```python
from build123d import *

# Parameters (mm, degrees)
SKETCH_1_R                = 45
EXTRUDE_2_DEPTH           = 25
SKETCH_2_R                = 35
CUT_EXTRUDE_1_DEPTH       = 4.5
SKETCH_3_R                = 27
CUT_EXTRUDE_2_DEPTH       = 8
SKETCH_4_R                = 18
CUT_EXTRUDE_3_DEPTH       = 8.5
SKETCH_10_R               = 42.5
CUT_EXTRUDE_5_DEPTH       = 4
HOLE_WIZARD_2_D           = 3.6
HOLE_WIZARD_2_CBORE_D     = 6
HOLE_WIZARD_2_CBORE_DEPTH = 3.4
PATTERN_CIRCULAR_2_COUNT  = 12
PATTERN_CIRCULAR_3_COUNT  = 8


with BuildPart() as part:
    # Sketch 1 → Extrude 2 (new body)
    with BuildSketch(Plane.XY):
        Circle(SKETCH_1_R)
    extrude(amount=EXTRUDE_2_DEPTH)

    # Sketch 2 → Cut-Extrude 1 (cut)
    with BuildSketch(Plane.XY.offset(25)):
        Circle(SKETCH_2_R)
    extrude(amount=-CUT_EXTRUDE_1_DEPTH, mode=Mode.SUBTRACT)

    # Sketch 3 → Cut-Extrude 2 (cut)
    with BuildSketch(Plane.XY.offset(20.5)):
        Circle(SKETCH_3_R)
    extrude(amount=-CUT_EXTRUDE_2_DEPTH, mode=Mode.SUBTRACT)

    # Sketch 4 → Cut-Extrude 3 (cut)
    with BuildSketch(Plane.XY.offset(12.5)):
        Circle(SKETCH_4_R)
    extrude(amount=-CUT_EXTRUDE_3_DEPTH, mode=Mode.SUBTRACT)

    # Sketch 10 → Cut-Extrude 5 (cut)
    with BuildSketch(Plane(origin=(0, 0, 0), x_dir=(-1, 0, 0), z_dir=(0, 0, -1))):
        Circle(SKETCH_10_R)
    extrude(amount=-CUT_EXTRUDE_5_DEPTH, mode=Mode.SUBTRACT)

    # Hole Wizard 2 (through all)
    with Locations(Plane(origin=(0, 0, 4), x_dir=(-1, 0, 0), z_dir=(0, 0, -1))):
        with Locations((0, 22)):
            hole_wizard_2 = CounterBoreHole(HOLE_WIZARD_2_D / 2, HOLE_WIZARD_2_CBORE_D / 2, HOLE_WIZARD_2_CBORE_DEPTH)

    # Pattern Circular 2: Hole Wizard 2 ×12 about axis
    pattern_circular_2_axis = Axis((0, 0, 0), (0, 0, 1))
    for i in range(1, PATTERN_CIRCULAR_2_COUNT):
        add(hole_wizard_2.rotate(pattern_circular_2_axis, i * 360 / PATTERN_CIRCULAR_2_COUNT), mode=Mode.SUBTRACT)

    # Sketch 17 → Hole Wizard M3 _1 (revolve, cut)
    with BuildSketch(Plane(origin=(0, 37.5, 4), x_dir=(0, 1, 0), z_dir=(1, 0, 0))):
        Polygon((0, 0), (0, 7.251075774), (1.25, 6.5), (1.25, 0), align=None)
    hole_wizard_m3_1 = revolve(axis=Axis((0, 37.5, -2.35), (0, 0, 1)), mode=Mode.SUBTRACT)

    # Pattern Circular 3: Hole Wizard M3 _1 ×8 about axis
    pattern_circular_3_axis = Axis((0, 0, 0), (0, 0, 1))
    for i in range(1, PATTERN_CIRCULAR_3_COUNT):
        add(hole_wizard_m3_1.rotate(pattern_circular_3_axis, i * 360 / PATTERN_CIRCULAR_3_COUNT), mode=Mode.SUBTRACT)


solid = part.part
```
Here's how the part is built. I have some questions about the finished solid (model axes, mm). A direction names the side the tool comes from. Coordinates: 2 decimals unless noted, no trailing zeros. Order: outer loops, then holes, each group sorted by start corner. A loop starts at its lowest first (then second) coordinate and runs counter-clockwise, first axis right, second up. Notation, with made-up numbers: (67, 56) - (122, 56) arc R11 ccw to (122, 77) - close; hole circle Ø2 at (85, -34.5). An arc over 180 degrees is marked (long way). One line per question, with ' | ' between items. Start each with the question number.
1. Please list where these lines run through material, in increasing order: line 1 along Y through (x, z) = (0, 5.95); line 2 along Z through (x, y) = (30, -5); line 3 along Y through (x, z) = (13, 10.5). Write a range as [from, to].
2. If we section it at B-B (y = 31): Write out the boundary of the cut face in (x, z).
3. I'm going to push flat-ended pins straight in: pin 1 Ø1.8 at (x, y) = (-19.5, 10.5) entering from -Z; pin 2 Ø6 at (x, z) = (1.5, 20) entering from +Y; pin 3 Ø6 at (x, y) = (-22, 0) entering from +Z; pin 4 Ø8 at (x, y) = (0, 22) entering from -Z. Where does each tip first touch, or does it pass through?
4. If we section it at C-C (x = 11): Give the number of separate pieces and of enclosed holes in the cut face, and give its area (3 significant figures).
5. If we mould it in two halves opening along X, with no side actions, what happens to faces 4 (the flat face through (23.1, -26.5, 25)), 5 (the cylindrical face through (-17.73, 9.78, 9.99)), 6 (the cylindrical face through (20.765, -39.923, 12.325)), 7 (the cylindrical face through (-27.094, -27.625, 7.204))? For each: released by +X, released by -X, zero draft, split by the parting line, or undercut.
6. Which directions (+Z, -Z, +X, -X, +Y, -Y) give clear straight access to the entire face, cutting with the end or side of a thin tool? Please do faces 1 (the flat face through (-0.4, 18.4, 12.5)), 2 (the cylindrical face through (8.972, -16.841, 5.676)), 3 (the cylindrical face through (-17.39, -11.69, 9.99)).
7. If we section it at A-A (z = 18.75): Write out the boundary of the cut face in (x, y).
Model answer:
1) line 1: y = [-45, -38.75], [-36.25, -25], [-19, -18], [18, 19], [25, 36.25], [38.75, 45] | line 2: z = [4, 20.5] | line 3: y = [-43.08, -12.45], [12.45, 43.08]
2) outline: (-32.62, 0) - (-29.07, 0) - (-29.07, 4) - (29.07, 4) - (29.07, 0) - (32.62, 0) - (32.62, 25) - (16.25, 25) - (16.25, 20.5) - (-16.25, 20.5) - (-16.25, 25) - (-32.62, 25) - close
3) pin 1: passes through | pin 2: stops at y = 45 | pin 3: stops at z = 12.5 | pin 4: stops at z = 4
4) separate pieces: 4 | enclosed holes: 0 | area: 840 mm²
5) face 4: zero draft | face 5: undercut | face 6: split by the parting line | face 7: undercut
6) face 1: +Z | face 2: -Z | face 3: +Z, -Z
7) outline: circle Ø90 at (0, 0); hole circle Ø54 at (0, 0)
